```python
from build123d import *

# Parameters (mm, degrees)
BOSS_EXTRUDE1_DEPTH = 63.3
FILLET4_R           = 3
FILLET5_R           = 25


with BuildPart() as part:
    # Sketch1 → Boss-Extrude1 (new body)
    with BuildSketch(Plane.XY):
        Polygon((0, 7), (7, 7), (7, 18.10712891), (7, 103.1), (13.8, 103.1), (13.8, 18.10712891), (13.8, 7), (20.8, 7), (20.8, 0), (0, 0), align=None)
    extrude(amount=BOSS_EXTRUDE1_DEPTH)

    # Fillet4
    fillet4_edges = [part.edges().sort_by_distance(p)[0] for p in [
        (10.4, 103.1, 0),
    ]]
    fillet(fillet4_edges, radius=FILLET4_R)

    # Fillet5
    fillet5_edges = [part.edges().sort_by_distance(p)[0] for p in [
        (10.4, 103.1, 63.3),
    ]]
    fillet(fillet5_edges, radius=FILLET5_R)


solid = part.part
```
For this review, take the finished solid that the model builds, in its own axes (mm). A direction names the side the tool comes from. Coordinates: 2 decimals unless noted, no trailing zeros. Loops run counter-clockwise (first coordinate to the right, second up) from the corner with the lowest first, then second, coordinate; pieces in that order, holes last. Notation, with made-up numbers: (-24.5, -16.75) -> (25.5, -16.75) arc R12 cw to (25.5, 0.25) -> close; hole circle Ø4 at (41, 42). An arc over 180 degrees is marked (long way). Return JSON: item names as keys, results as strings. Group by question number.
(1) Consider section D-D, the plane x = 12.25. Give the boundary of the cut face in (y, z).
(2) Tool access review of faces 1 (the flat face through (0, 3, 31)), 2 (the flat face through (17, 7, 31)), 3 (the flat face through (7, 56, 31)): name each direction out of +Z, -Z, +X, -X, +Y, -Y from which nothing blocks a thin tool from reaching the whole face with its end or side.
(3) Consider section B-B, the plane x = 2.5. Give the boundary of the cut face in (y, z).
(4) For pin 1 Ø2 at (x, z) = (16, 41.5) entering from +Y; pin 2 Ø5 at (y, z) = (51, 13.5) entering from +X; pin 3 Ø10 at (x, z) = (3, 19) entering from +Y; pin 4 Ø5 at (y, z) = (50, 28.5) entering from -X, all flat-tipped, find the tip position at first contact; note any pin that passes through.
(5) Consider section C-C, the plane y = 69. Give the boundary of the cut face in (x, z), plus the area to 3 significant figures.
(6) Consider section A-A, the plane z = 6.5. Give the boundary of the cut face in (x, y), plus the area to 3 significant figures.
(7) To check wall thickness, follow L1, parallel to Y at x = 3.5, z = 17.5; L2, parallel to X at y = 16.5, z = 48.5; L3, parallel to Y at x = 10.25, z = 45.5. State the ranges of each line that lie inside material, in increasing order.
Results below:
{
 "1": {"outline": "(0, 0) -> (100.1, 0) arc R3 ccw to (103.1, 3) -> (103.1, 38.3) arc R25 ccw to (78.1, 63.3) -> (0, 63.3) -> close"},
 "2": {"face 1": "+Z, -Z, -X, +Y, -Y", "face 2": "+Z, -Z, +X, +Y", "face 3": "+Z, -Z, -X, +Y"},
 "3": {"outline": "(0, 0) -> (7, 0) -> (7, 63.3) -> (0, 63.3) -> close"},
 "4": {"pin 1": "stops at y = 7", "pin 2": "stops at x = 13.8", "pin 3": "stops at y = 103.1", "pin 4": "stops at x = 7"},
 "5": {"outline": "(7, 0) -> (13.8, 0) -> (13.8, 63.3) -> (7, 63.3) -> close", "area": "430 mm2"},
 "6": {"outline": "(0, 0) -> (20.8, 0) -> (20.8, 7) -> (13.8, 7) -> (13.8, 103.1) -> (7, 103.1) -> (7, 7) -> (0, 7) -> close", "area": "799 mm2"},
 "7": {"L1": "y = 0 to 7", "L2": "x = 7 to 13.8", "L3": "y = 0 to 102.04"}
}
